Could you check a few things on this drawing? It's one solid part, dimensions in mm from its lowest x, y, z. A direction names the side the tool comes from. Give positions to 0.01 mm unless a question says otherwise; leave off trailing zeros. Order: outer loops, then holes, each group sorted by start corner. A loop starts at its lowest first (then second) coordinate and runs counter-clockwise, first axis right, second up.
(1) On a 3-axis mill with a long thin cutter (end or side, diameter ignored), from which of +Z, -Z, +X, -X, +Y, -Y can I reach the whole of each face in a straight line? I mean the marked faces 1 and 2. Say none if no direction works.
(2) Will these pins go through, and if not, where does the flat tip stop? pin 1 (4 mm diameter, centred on x = 4, y = 2.5, fed in from +Z); pin 2 (1 mm diameter, centred on x = 2.5, y = 1.5, fed in from +Z); pin 3 (1.5 mm diameter, centred on y = 6, z = 11, fed in from -X).
(3) Imagine slicing it at B-B, the plane y = 3.25. Write out the boundary of the cut face in (x, z), then the cut area to 3 significant figures.
(4) Imagine slicing it at C-C, the plane x = 10.5. Write out the boundary of the cut face in (y, z), then the cut area to 3 significant figures.
(5) Imagine slicing it at D-D, the plane z = 19.5. Write out the boundary of the cut face in (x, y).
(6) If I drill on probe 1 along Y at (x, z) = (6.5, 24.5); probe 2 along Y at (x, z) = (5.75, 13); probe 3 along X at (y, z) = (4.5, 3.5), over which ranges is the centre line in solid material (lowest first)?
(7) Imagine slicing it at A-A, the plane z = 6.5. Write out the boundary of the cut face in (x, y), then the cut area to 4 significant figures.
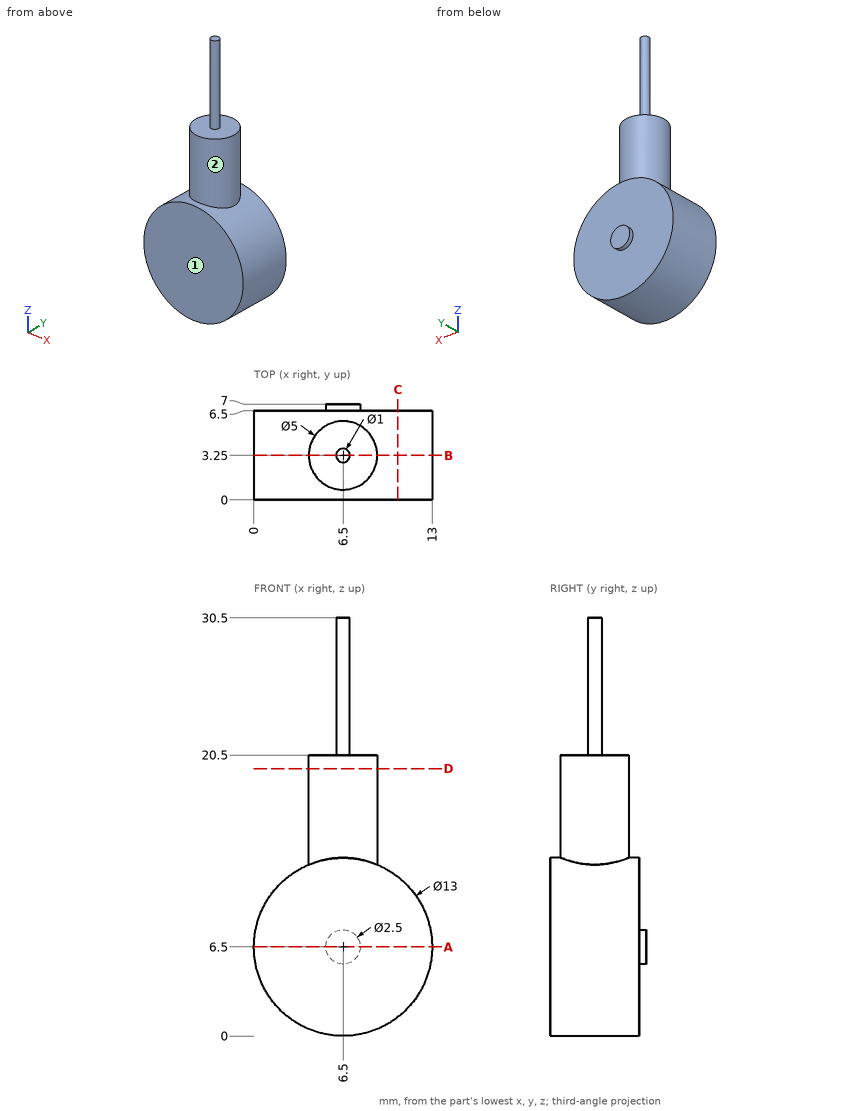
Answer block:
1. face 1: +Z, -Z, +X, -X, -Y
1. face 2: +Z
2. pin 1: stops at z = 20.5
2. pin 2: stops at z = 11.98
2. pin 3: stops at x = 1.19
3. outline: (4, 12.5) arc R6.5 ccw (long way) to (9, 12.5) - (9, 20.5) - (7, 20.5) - (7, 30.5) - (6, 30.5) - (6, 20.5) - (4, 20.5) - close
3. area: 181 mm2
4. outline: (0, 1.38) - (6.5, 1.38) - (6.5, 11.62) - (0, 11.62) - close
4. area: 66.6 mm2
5. outline: circle Ø5 at (6.5, 3.25)
6. probe 1: y = 2.75 to 3.75
6. probe 2: y = 0.87 to 5.63
6. probe 3: x = 0.73 to 12.27
7. outline: (0, 0) - (13, 0) - (13, 6.5) - (7.75, 6.5) - (7.75, 7) - (5.25, 7) - (5.25, 6.5) - (0, 6.5) - close
7. area: 85.75 mm2
